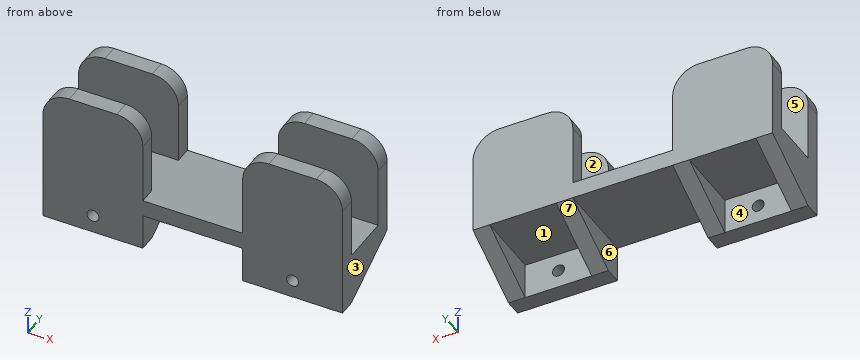
from build123d import *

# Parameters (mm, degrees)
SKETCH1_W           = 114.3
SKETCH1_H           = 19.05
BOSS_EXTRUDE1_DEPTH = 6.35
SKETCH3_W           = 38.1
SKETCH3_H           = 33.02
SKETCH3_W_2         = 114.3
SKETCH3_H_2         = 13.716
SKETCH3_H_3         = 6.35
BOSS_EXTRUDE2_DEPTH = 6.35
SKETCH4_W           = 38.1
SKETCH4_H           = 33.02
BOSS_EXTRUDE3_DEPTH = 6.35
SKETCH6_W           = 38.1
SKETCH6_H           = 13.716
CUT_EXTRUDE1_DEPTH  = 74.900469552
BOSS_EXTRUDE4_DEPTH = 6.35
BOSS_EXTRUDE5_DEPTH = 6.35
BOSS_EXTRUDE6_DEPTH = 6.35
BOSS_EXTRUDE7_DEPTH = 6.35
SKETCH10_R          = 2.286
CUT_EXTRUDE2_DEPTH  = 74.900469552
FILLET2_R           = 10


with BuildPart() as part:
    # Sketch1 → Boss-Extrude1 (new body)
    with BuildSketch(Plane.XY):
        Rectangle(SKETCH1_W, SKETCH1_H)
    extrude(amount=BOSS_EXTRUDE1_DEPTH)

    # Sketch3 → Boss-Extrude2 (add)
    with BuildSketch(Plane(origin=(0, -9.525, 0), x_dir=(-1, 0, 0), z_dir=(0, -1, 0))):
        with Locations((38.1, -22.86)):
            Rectangle(SKETCH3_W, SKETCH3_H)
        with Locations((0, 6.858)):
            Rectangle(SKETCH3_W_2, SKETCH3_H_2)
        with Locations((0, -3.175)):
            Rectangle(SKETCH3_W_2, SKETCH3_H_3)
        with Locations((-38.1, -22.86)):
            Rectangle(SKETCH3_W, SKETCH3_H)
    extrude(amount=BOSS_EXTRUDE2_DEPTH)

    # Sketch4 → Boss-Extrude3 (add)
    with BuildSketch(Plane(origin=(0, 9.525, 0), x_dir=(1, 0, 0), z_dir=(0, 1, 0))):
        with Locations((38.1, -22.86)):
            Rectangle(SKETCH4_W, SKETCH4_H)
        Polygon((57.15, -6.35), (57.15, 0), (-57.15, 0), (-57.15, -6.35), (-19.05, -6.35), (19.05, -6.35), align=None)
        with Locations((-38.1, -22.86)):
            Rectangle(SKETCH4_W, SKETCH4_H)
    extrude(amount=BOSS_EXTRUDE3_DEPTH)

    # Sketch6 → Cut-Extrude1 (cut, through all)
    with BuildSketch(Plane(origin=(0, -9.525, 0), x_dir=(1, 0, 0), z_dir=(0, 1, 0))):
        with Locations((0, 6.858)):
            Rectangle(SKETCH6_W, SKETCH6_H)
    extrude(amount=-CUT_EXTRUDE1_DEPTH, mode=Mode.SUBTRACT)

    # Sketch5 → Boss-Extrude4 (add)
    with BuildSketch(Plane(origin=(57.15, 0, 0), x_dir=(0, 0, -1), z_dir=(1, 0, 0))):
        Polygon((13.716, -9.525), (0, 15.875), (0, -9.525), align=None)
    extrude(amount=-BOSS_EXTRUDE4_DEPTH)

    # Sketch7 → Boss-Extrude5 (add)
    with BuildSketch(Plane.ZY.offset(-19.05)):
        Polygon((-13.716, -9.525), (0, -9.525), (0, 15.875), align=None)
    extrude(amount=-BOSS_EXTRUDE5_DEPTH)

    # Sketch8 → Boss-Extrude6 (add)
    with BuildSketch(Plane(origin=(-19.05, 0, 0), x_dir=(0, 0, -1), z_dir=(1, 0, 0))):
        Polygon((13.716, -9.525), (0, 15.875), (0, -9.525), align=None)
    extrude(amount=-BOSS_EXTRUDE6_DEPTH)

    # Sketch9 → Boss-Extrude7 (add)
    with BuildSketch(Plane.ZY.offset(57.15)):
        Polygon((-13.716, -9.525), (0, -9.525), (0, 15.875), align=None)
    extrude(amount=-BOSS_EXTRUDE7_DEPTH)

    # Sketch10 → Cut-Extrude2 (cut, through all)
    with BuildSketch(Plane(origin=(0, -9.525, 0), x_dir=(1, 0, 0), z_dir=(0, 1, 0))):
        with Locations(Location((38.1, 6.858, 0), (0, 0, 270))):
            Circle(SKETCH10_R)
        with Locations(Location((-38.1, 6.858, 0), (0, 0, 270))):
            Circle(SKETCH10_R)
    extrude(amount=-CUT_EXTRUDE2_DEPTH, mode=Mode.SUBTRACT)

    # Fillet2
    fillet2_edges = [part.edges().sort_by_distance(p)[0] for p in [
        (-19.05, -12.7, 39.37),
        (-57.15, -12.7, 39.37),
        (57.15, -12.7, 39.37),
        (19.05, -12.7, 39.37),
        (19.05, 12.7, 39.37),
        (57.15, 12.7, 39.37),
        (-57.15, 12.7, 39.37),
        (-19.05, 12.7, 39.37),
    ]]
    fillet(fillet2_edges, radius=FILLET2_R)


solid = part.part
For this review, take the finished solid that the model builds, in its own axes (mm). Face numbers are marked on the shaded views. A direction names the side the tool comes from. Coordinates: 2 decimals unless noted, no trailing zeros. Loops run counter-clockwise (first coordinate to the right, second up) from the corner with the lowest first, then second, coordinate; pieces in that order, holes last. Notation, with made-up numbers: (-33, 13.25) - (-14, 13.25) arc R16 cw to (-14, 40.25) - close; hole circle Ø9 at (-34, 39.5). An arc over 180 degrees is marked (long way). Return JSON: item names as keys, results as strings.
Item 1: Take a section at C-C (z = 32.5). Give the boundary of the cut face in (x, y) (3 decimals), then the cut area to 3 significant figures.
Determined:
{"outline": "(-56.648, -15.875) - (-19.552, -15.875) - (-19.552, -9.525) - (-56.648, -9.525) - close; (-56.648, 9.525) - (-19.552, 9.525) - (-19.552, 15.875) - (-56.648, 15.875) - close; (19.552, -15.875) - (56.648, -15.875) - (56.648, -9.525) - (19.552, -9.525) - close; (19.552, 9.525) - (56.648, 9.525) - (56.648, 15.875) - (19.552, 15.875) - close", "area": "942 mm2"}
Item 2: For line 1 (X direction, y = -9, z = -10); line 2 (Y direction, x = -23.5, z = 15.5) (3 decimals); line 3 (X direction, y = -14, z = -11), list the stretches that pass through material, from the lowest coordinate up.
Determined:
{"line 1": "x = -57.15 to -50.8, -25.4 to -19.05, 19.05 to 25.4, 50.8 to 57.15", "line 2": "y = -15.875 to -9.525, 9.525 to 15.875", "line 3": "x = -57.15 to -19.05, 19.05 to 57.15"}
Item 3: Take a section at D-D (y = -8). Give the boundary of the cut face in (x, z), then the cut area to 3 significant figures.
Determined:
{"outline": "(-57.15, -12.89) - (-50.8, -12.89) - (-50.8, 0) - (-25.4, 0) - (-25.4, -12.89) - (-19.05, -12.89) - (-19.05, 0) - (19.05, 0) - (19.05, -12.89) - (25.4, -12.89) - (25.4, 0) - (50.8, 0) - (50.8, -12.89) - (57.15, -12.89) - (57.15, 6.35) - (-57.15, 6.35) - close", "area": "1,050 mm2"}
Item 4: Insertion check: pin 1 (3 mm diameter, centred on x = -44, y = 3.5, fed in from -Z); pin 2 (4 mm diameter, centred on x = 37.5, z = -6, fed in from +Y) (3 decimals). Each pin has a flat end and moves straight along its axis. Give the tip position at first contact, or say it passes through.
Determined:
{"pin 1": "stops at z = 0", "pin 2": "stops at y = -9.525"}
Item 5: Take a section at B-B (x = 38.1). Give the boundary of the cut face in (y, z) (3 decimals), then the cut area to 3 significant figures.
Determined:
{"outline": "(-15.875, -13.716) - (-9.525, -13.716) - (-9.525, -9.144) - (-15.875, -9.144) - close; (-15.875, -4.572) - (-9.525, -4.572) - (-9.525, 0) - (15.875, 0) - (15.875, 39.37) - (9.525, 39.37) - (9.525, 6.35) - (-9.525, 6.35) - (-9.525, 39.37) - (-15.875, 39.37) - close", "area": "679 mm2"}
Item 6: Take a section at A-A (y = -13). Give the boundary of the cut face in (x, z).
Determined:
{"outline": "(-57.15, -13.72) - (-19.05, -13.72) - (-19.05, 0) - (19.05, 0) - (19.05, -13.72) - (57.15, -13.72) - (57.15, 29.37) arc R10 ccw to (47.15, 39.37) - (29.05, 39.37) arc R10 ccw to (19.05, 29.37) - (19.05, 6.35) - (-19.05, 6.35) - (-19.05, 29.37) arc R10 ccw to (-29.05, 39.37) - (-47.15, 39.37) arc R10 ccw to (-57.15, 29.37) - close; hole circle Ø4.57 at (-38.1, -6.86); hole circle Ø4.57 at (38.1, -6.86)"}
Item 7: Mouldability with a two-part tool opening along X and no side actions: class the marked faces 1, 2 and 3 as pulls with the +X half, pulls with the -X half, needs draft (parallel to the pull), parting line crosses it, or undercut.
Determined:
{"face 1": "undercut", "face 2": "needs draft", "face 3": "pulls with the +X half"}
Item 8: For the marked faces 4, 5, 6 and 7, list the 3-axis set-ups (+Z, -Z, +X, -X, +Y, -Y) from which the entire face can be reached by the end or side of a thin tool; tool diameter is ignored.
Determined:
{"face 4": "-Z, +Y", "face 5": "+Z, +X, -X", "face 6": "-Z, +Y, -Y", "face 7": "-Z, +X, -X, +Y"}
